Can you work these out from the model? Positions are in its coordinate system, mm. Face numbers are marked on the shaded views. A direction names the side the tool comes from. Give positions to 0.01 mm unless a question says otherwise; leave off trailing zeros. Write each loop counter-clockwise with the first axis right and the second up, starting at its lowest first coordinate (ties: lowest second). Pieces come first, ordered by that corner, then holes. Notation, with made-up numbers: (39, -22) - (93, -22) arc R34 ccw to (93, 10) - close; hole circle Ø6 at (7.25, 49). An arc over 180 degrees is marked (long way). Return JSON: item names as keys, results as strings. Group by question number.
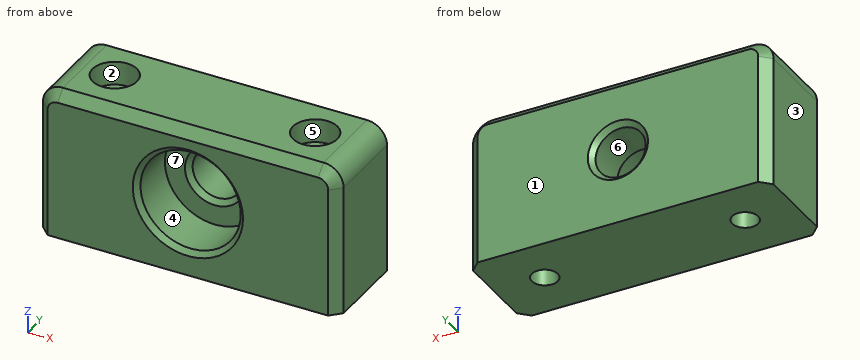
from build123d import *

# Parameters (mm, degrees)
F0_W           = 76.2
F0_H           = 38.1
F1_DEPTH       = 25.4
F2_R           = 5.08
F3_R           = 12.7
F4_DEPTH       = 12.7
F5_R           = 6.35
F6_DEPTH       = 12.701
F8_D           = 6.6
F8_CBORE_D     = 11.25
F8_CBORE_DEPTH = 6
F9_SIZE        = 2.54
F10_SIZE       = 1.27


with BuildPart() as f1:
    # F0 (on Front) → F1 (new body)
    with BuildSketch(Plane.XZ):
        with Locations((38.1, 19.05)):
            Rectangle(F0_W, F0_H)
    extrude(amount=F1_DEPTH)

    # F2
    f2_edges = [f1.edges().sort_by_distance(p)[0] for p in [
        (76.2, -12.7, 38.1),
        (0, -12.7, 38.1),
    ]]
    fillet(f2_edges, radius=F2_R)

    # F3 (on face) → F4 (cut)
    with BuildSketch(Plane.XZ.offset(25.4)):
        with Locations((38.1, 19.05)):
            Circle(F3_R)
    extrude(amount=-F4_DEPTH, mode=Mode.SUBTRACT)

    # F5 (on face) → F6 (cut, through all)
    with BuildSketch(Plane.XZ.offset(12.7)):
        with Locations((38.1, 19.05)):
            Circle(F5_R)
    extrude(amount=-F6_DEPTH, mode=Mode.SUBTRACT)

    # F8 (through all)
    with Locations(Plane.XY.offset(38.1)):
        with Locations((12.7, -12.7), (63.5, -12.7)):
            CounterBoreHole(F8_D / 2, F8_CBORE_D / 2, F8_CBORE_DEPTH)

    # F9
    f9_edges = [f1.edges().sort_by_distance(p)[0] for p in [
        (38.1, -25.4, 38.1),
        (38.1, 0, 38.1),
    ]]
    chamfer(f9_edges, length=F9_SIZE)

    # F10
    f10_edges = [f1.edges().sort_by_distance(p)[0] for p in [
        (31.75, 0, 19.05),
        (31.75, -12.7, 19.05),
        (25.4, -25.4, 19.05),
    ]]
    chamfer(f10_edges, length=F10_SIZE)


solid = f1.part
1) On a 3-axis mill with a long thin cutter (end or side, diameter ignored), from which of +Z, -Z, +X, -X, +Y, -Y can I reach the whole of each face in a straight line? I mean the marked faces 5, 6 and 7. Say none if no direction works.
2) Imagine slicing it at D-D, the plane x = 38.1. Write out the boundary of the cut face in (y, z).
3) We'd pull the mould along X, two halves only. Please class the marked faces 1, 2, 3 and 4: pulls with the +X half, pulls with the -X half, needs draft (parallel to the pull), parting line crosses it, or undercut.
4) Imagine slicing it at B-B, the plane x = 12.7. Write out the boundary of the cut face in (y, z) (3 decimals).
5) I need wall thicknesses on line 1 along Z through (x, y) = (38.1, -19.25); line 2 along Y through (x, z) = (63.5, 34) (3 decimals); line 3 along Z through (x, y) = (15.5, -17.25). Which ranges of each line are inside material? Lowest first, please.
6) Will these pins go through, and if not, where does the flat tip stop? pin 1 Ø3.5 at (x, y) = (61, -13) entering from +Z; pin 2 Ø11.5 at (x, z) = (38.1, 19.05) entering from +Y.
7) Imagine slicing it at A-A, the plane z = 19.05. Write out the boundary of the cut face in (x, y).
8) Imagine slicing it at C-C, the plane y = -14.5. Write out the boundary of the cut face in (x, z), and give its area (3 significant figures).
Resolved:
{
 "1": {"face 5": "+Z", "face 6": "+Y, -Y", "face 7": "-Y"},
 "2": {"outline": "(-25.4, 0) - (0, 0) - (0, 11.43) - (-1.27, 12.7) - (-11.43, 12.7) - (-12.7, 11.43) - (-12.7, 6.35) - (-24.13, 6.35) - (-25.4, 5.08) - close; (-25.4, 33.02) - (-24.13, 31.75) - (-12.7, 31.75) - (-12.7, 26.67) - (-11.43, 25.4) - (-1.27, 25.4) - (0, 26.67) - (0, 35.56) - (-2.54, 38.1) - (-22.86, 38.1) - (-25.4, 35.56) - close"},
 "3": {"face 1": "needs draft", "face 2": "undercut", "face 3": "pulls with the -X half", "face 4": "undercut"},
 "4": {"outline": "(-25.4, 0) - (-16, 0) - (-16, 32.1) - (-18.325, 32.1) - (-18.325, 38.1) - (-22.86, 38.1) - (-25.4, 35.56) - close; (-9.4, 0) - (0, 0) - (0, 35.56) - (-2.54, 38.1) - (-7.075, 38.1) - (-7.075, 32.1) - (-9.4, 32.1) - close"},
 "5": {"line 1": "0 to 6.35, 31.75 to 38.1", "line 2": "-25.4 to -18.325, -7.075 to 0", "line 3": "0 to 32.1"},
 "6": {"pin 1": "z = 32.1", "pin 2": "through"},
 "7": {"outline": "(0, -22.86) - (2.54, -25.4) - (24.13, -25.4) - (25.4, -24.13) - (25.4, -12.7) - (30.48, -12.7) - (31.75, -11.43) - (31.75, -1.27) - (30.48, 0) - (2.54, 0) - (0, -2.54) - close; (44.45, -11.43) - (45.72, -12.7) - (50.8, -12.7) - (50.8, -24.13) - (52.07, -25.4) - (73.66, -25.4) - (76.2, -22.86) - (76.2, -2.54) - (73.66, 0) - (45.72, 0) - (44.45, -1.27) - close; hole circle Ø6.6 at (12.7, -12.7); hole circle Ø6.6 at (63.5, -12.7)"},
 "8": {"outline": "(0, 0) - (9.93, 0) - (9.93, 32.1) - (7.37, 32.1) - (7.37, 38.1) - (5.08, 38.1) arc R5.08 ccw to (0, 33.02) - close; (15.47, 0) - (60.73, 0) - (60.73, 32.1) - (58.17, 32.1) - (58.17, 38.1) - (18.03, 38.1) - (18.03, 32.1) - (15.47, 32.1) - close; (66.27, 0) - (76.2, 0) - (76.2, 33.02) arc R5.08 ccw to (71.12, 38.1) - (68.83, 38.1) - (68.83, 32.1) - (66.27, 32.1) - close; hole circle Ø25.4 at (38.1, 19.05)", "area": "1,900 mm^2"}
}
